Verification items for the finished model (mm, model axes). Face numbers are marked on the shaded views. Give positions to 0.01 mm unless a question says otherwise; leave off trailing zeros. Loops run counter-clockwise (first coordinate to the right, second up) from the corner with the lowest first, then second, coordinate; pieces in that order, holes last. Notation, with made-up numbers: (59, 8.5) -> (95, 8.5) arc R10 ccw to (95, 14.5) -> close; hole circle Ø7 at (76, 39.25). An arc over 180 degrees is marked (long way). Use one line per item in the form item = value. Start each with the question number.
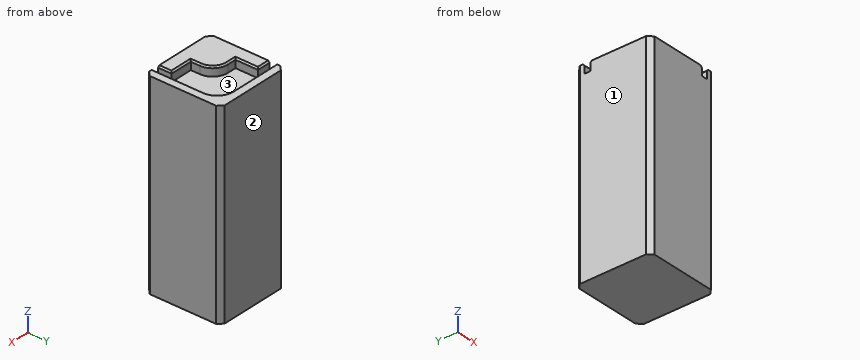
from build123d import *

# Parameters (mm, degrees)
SKETCH029_W     = 50
SKETCH029_H     = 50
PAD017_DEPTH    = 130
POCKET007_DEPTH = 6
CHAMFER006_SIZE = 1
CHAMFER007_SIZE = 3


with BuildPart() as part:
    # Sketch029 → Pad017 (new body)
    with BuildSketch(Plane.XY):
        Rectangle(SKETCH029_W, SKETCH029_H)
    extrude(amount=PAD017_DEPTH)

    # Sketch030 (on DatumPlane) → Pocket007 (cut)
    with BuildSketch(Plane.XY.offset(130)):
        with BuildLine():
            Line((-31, 19), (9, 19))
            ThreePointArc((19, 9), (16.071068, 16.071068), (9, 19))
            Line((19, 9), (19, -31))
            Line((15, -31), (19, -31))
            Line((15, -16), (15, -31))
            Line((15, -16), (0, -16))
            Line((0, -16), (0, -10))
            ThreePointArc((0, -10), (-2.928932, -2.928932), (-10, 0))
            Line((-10, 0), (-16, 0))
            Line((-16, 0), (-16, 15))
            Line((-16, 15), (-31, 15))
            Line((-31, 15), (-31, 19))
        make_face()
    extrude(amount=-POCKET007_DEPTH, mode=Mode.SUBTRACT)

    # Chamfer006
    chamfer006_edges = [part.edges().sort_by_distance(p)[0] for p in [
        (19, -8, 130),
        (-16, 7.5, 130),
        (-13, 0, 130),
        (7.5, -16, 130),
        (15, -20.5, 130),
        (-20.5, 15, 130),
    ]]
    chamfer(chamfer006_edges, length=CHAMFER006_SIZE)

    # Chamfer007
    chamfer007_edges = [part.edges().sort_by_distance(p)[0] for p in [
        (25, -25, 65),
        (-25, -25, 65),
        (25, 25, 65),
        (-25, 25, 65),
    ]]
    chamfer(chamfer007_edges, length=CHAMFER007_SIZE)


solid = part.part
Item 1: Draft check along X on the marked faces 1, 2 and 3. Enter one of: +X half, -X half, draft (parallel to the pull), parting line (faces both ways), or undercut.
Item 2: Sectioned sample at A-A, the plane y = 5. Enter the section's corners in (x, z), and give its area (3 significant figures).
Item 3: Material ranges on line 1 (Z direction, x = 11, y = 8); line 2 (Z direction, x = -1.5, y = -5), recorded low to high.
Outcome:
q1.face_1 = -X half
q1.face_2 = draft
q1.face_3 = undercut
q2.outline = (-25, 0) -> (25, 0) -> (25, 130) -> (20, 130) -> (19, 129) -> (19, 124) -> (-16, 124) -> (-16, 129) -> (-17, 130) -> (-25, 130) -> close
q2.area = 6,290 mm^2
q3.line_1 = 0 to 124
q3.line_2 = 0 to 129.14
